from build123d import *

# Parameters (mm, degrees)
F1_DEPTH = 19.05
F3_DEPTH = 9.525
F5_R     = 2.4892
F6_DEPTH = 25.4


# Not quite as in the source:
# - a length typed as a fraction of an inch, garbled in the dataset ("3 / 203.2 mm" for 3/8 in), is restored


with BuildPart() as f1:
    # F0 (on Front) → F1 (new body)
    with BuildSketch(Plane.XZ):
        with BuildLine():
            ThreePointArc((0, 18.6436), (12.9107977631, 13.4497257251), (18.6280212841, 0.762))
            Line((18.6280212841, 0.762), (28.7880212841, 0.762))
            Line((28.7880212841, 0.762), (28.7880212841, 5.842))
            Line((28.7880212841, 5.842), (20.3621203454, 5.842))
            ThreePointArc((20.3621203454, 5.842), (12.7473588982, 16.9189169299), (0, 21.1836))
            Line((0, 21.1836), (0, 18.6436))
        make_face()
    extrude(amount=F1_DEPTH)

    # F2 (on face) → F3 (cut)
    with BuildSketch(Plane(origin=(0, 0, 0), x_dir=(-1, 0, 0), z_dir=(0, 1, 0))):
        with BuildLine():
            ThreePointArc((0, 19.8755), (-14.0541008295, 14.0541008295), (-19.8755, 0))
            Line((-19.8755, 0), (0, 0))
            Line((0, 0), (0, 19.8755))
        make_face()
    extrude(amount=-F3_DEPTH, mode=Mode.SUBTRACT)

    # F4: F1 across face


with BuildPart() as f1_1:
    add(f1.part)
    add(f1.part.mirror(Plane(origin=(0, -11.0496287129, 20.1229823432), x_dir=(0, -1, 0), z_dir=(-1, 0, 0))))

    # F5 (on Top) → F6 (cut)
    with BuildSketch(Plane.XY):
        with Locations((0, -15.875)):
            Circle(F5_R)
        with Locations((0, -3.175)):
            Circle(F5_R)
        with Locations((-25.6130212841, -9.525)):
            Circle(F5_R)
        with Locations((25.6130212841, -9.525)):
            Circle(F5_R)
    extrude(amount=F6_DEPTH, mode=Mode.SUBTRACT)


solid = f1_1.part
The model under review builds one solid part; all positions refer to its coordinate system, in mm. A direction names the side the tool comes from. Give positions to 0.01 mm unless a question says otherwise; leave off trailing zeros. Order: outer loops, then holes, each group sorted by start corner. A loop starts at its lowest first (then second) coordinate and runs counter-clockwise, first axis right, second up. Notation, with made-up numbers: M 17.25,-32.5 L 66.25,-32.5 A8 ccw 66.25,-22.5 Z; hole C 12.5,9.25 d3. An arc over 180 degrees is marked long. Answer in a Markdown table with one row per item. Add a question column.
1. For pin 1 Ø4 at (x, y) = (7.5, -14.5) entering from -Z; pin 2 Ø2.5 at (x, y) = (-24, -9) entering from +Z; pin 3 Ø8 at (x, y) = (20.5, -11) entering from +Z, all flat-tipped, find the tip position at first contact; note any pin that passes through.
2. Machinability: for faces 1 (the flat face through (-23, -9, 5.842)), 2 (the cylindrical face through (-27.59, -11.04, 3.27)), 3 (the flat face through (0, -9.525, 19)), which of the approach directions +Z, -Z, +X, -X, +Y, -Y give a long, thin tool a straight path to every point of the face, cutting with its end or side? Answer none if there is none.
3. Add section B-B on y = -17.25. State the section outline as (x, z) points, plus the area to 3 significant figures.
4. Add section A-A on z = 3.5. State the section outline as (x, y) points (3 decimals).
5. Mouldability with a two-part tool opening along X and no side actions: class faces 4 (the flat face through (28.788, -9, 3)), 5 (the cylindrical face through (23.64, -11.04, 3.27)), 6 (the flat face through (23, -9, 5.842)) as released by +X, released by -X, zero draft, split by the parting line, or undercut.
6. Add section C-C on z = 9.75. State the section outline as (x, y) points (3 decimals), plus the area to 3 significant figures.
7. To check wall thickness, follow line 1 along Y through (x, z) = (0, 20.25); line 2 along X through (y, z) = (-3.25, 12.5); line 3 along Z through (x, y) = (-25, -5). State the ranges of each line that lie inside material, in increasing order.
The answers:
| question | item | result |
|---|---|---|
| 1 | pin 1 | z = 16.04 |
| 1 | pin 2 | z = 5.84 |
| 1 | pin 3 | z = 13.29 |
| 2 | face 1 | +Z, -X, +Y, -Y |
| 2 | face 2 | +Z, -Z |
| 2 | face 3 | -Z, +Y |
| 3 | outline | M -28.79,0.76 L -18.63,0.76 A18.64 cw -2.07,18.53 L -2.07,21.08 A21.18 ccw -20.36,5.84 L -28.79,5.84 Z; M 2.07,18.53 A18.64 cw 18.63,0.76 L 28.79,0.76 L 28.79,5.84 L 20.36,5.84 A21.18 ccw 2.07,21.08 Z |
| 3 | area | 225 mm2 |
| 4 | outline | M -28.788,-19.05 L -18.312,-19.05 L -18.312,-9.525 L -19.565,-9.525 L -19.565,0 L -28.788,0 Z; M 18.312,-19.05 L 28.788,-19.05 L 28.788,0 L 19.565,0 L 19.565,-9.525 L 18.312,-9.525 Z; hole C -25.613,-9.525 d4.978; hole C 25.613,-9.525 d4.978 |
| 5 | face 4 | released by +X |
| 5 | face 5 | undercut |
| 5 | face 6 | zero draft |
| 6 | outline | M -18.806,-19.05 L -15.891,-19.05 L -15.891,-9.525 L -17.32,-9.525 L -17.32,0 L -18.806,0 Z; M 15.891,-19.05 L 18.806,-19.05 L 18.806,0 L 17.32,0 L 17.32,-9.525 L 15.891,-9.525 Z |
| 6 | area | 83.9 mm2 |
| 7 | line 1 | -19.05 to -18.36, -13.39 to -5.66, -0.69 to 0 |
| 7 | line 2 | -17.1 to -15.45, 15.45 to 17.1 |
| 7 | line 3 | 0.76 to 5.84 |
